Can you work these out from the drawing? Everything is in mm from the part's minimum corner. A direction names the side the tool comes from. Round coordinates to 2 decimals unless told otherwise and drop trailing zeros. Order: outer loops, then holes, each group sorted by start corner. A loop starts at its lowest first (then second) coordinate and runs counter-clockwise, first axis right, second up. Notation, with made-up numbers: (13.25, 83.25) -> (43.25, 83.25) arc R31 cw to (43.25, 119.25) -> close; hole circle Ø8 at (-31, 89). An arc over 180 degrees is marked (long way). One line per item, written item: value.
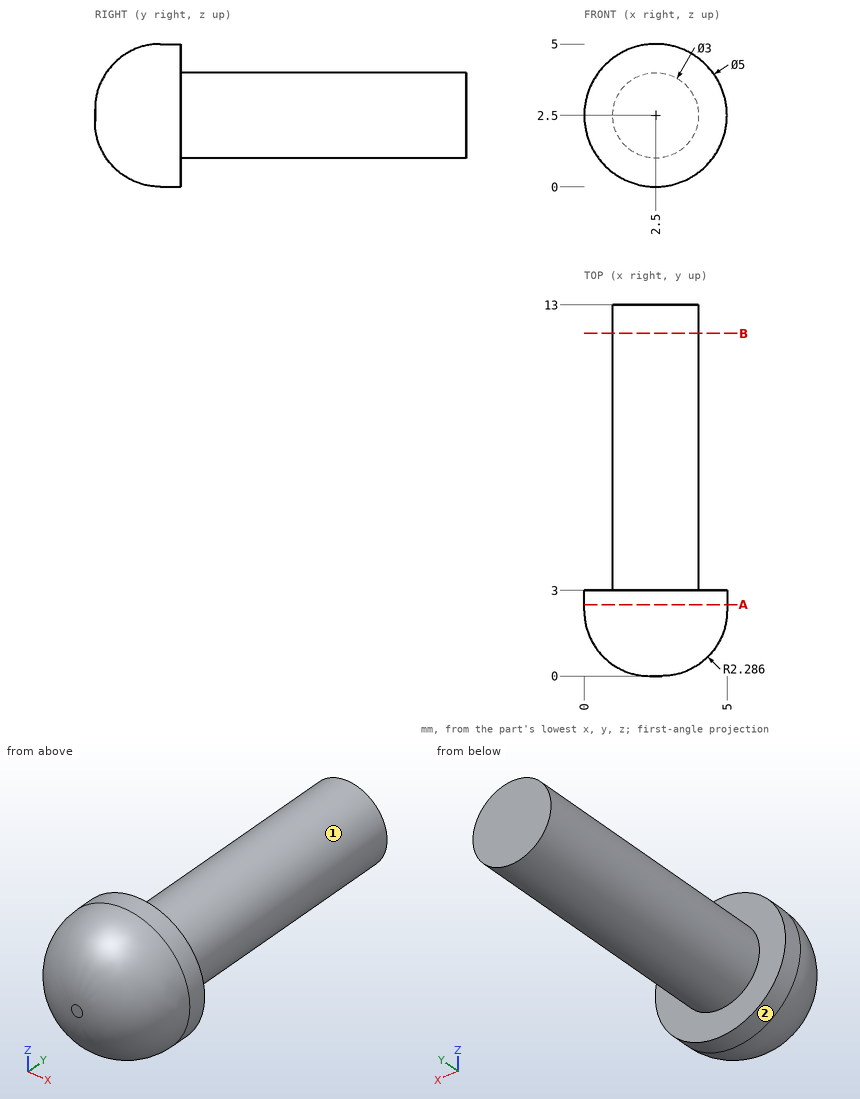
Q1. I want a section at B-B on y = 12. Write out the boundary of the cut face in (x, z).
Answers:
outline: circle Ø3 at (2.5, 2.5)
Q2. I need wall thicknesses on line 1 along Z through (x, y) = (2.45, 7.75); line 2 along X through (y, z) = (2.75, 2.6); line 3 along Y through (x, z) = (3.15, 4.5). Which ranges of each line are inside material? Lowest first, please.
Answers:
line 1: 1 to 4
line 2: 0 to 5
line 3: 1 to 3
Q3. For P1, Ø3, axis at x = 2, z = 4, coming from the +Y side; P2, Ø1, axis at x = 1, y = 1.5, coming from the -Z side; P3, Ø3, axis at x = 2.5, y = 10, coming from the +Z side, each with a flat end and sliding along its axis, tell me the tip position at first contact or that it passes through.
Answers:
P1: y = 13
P2: z = 0.31
P3: z = 4
Q4. Which directions (+Z, -Z, +X, -X, +Y, -Y) give clear straight access to the entire face, cutting with the end or side of a thin tool? Please do the marked faces 1 and 2.
Answers:
face 1: +Y
face 2: +Y, -Y
Q5. I want a section at A-A on y = 2.5. Write out the boundary of the cut face in (x, z).
Answers:
outline: circle Ø5 at (2.5, 2.5)
